CAD build for the part. Positions are in the model's coordinates, mm. A direction names the side the tool comes from. Round coordinates to 2 decimals unless told otherwise and drop trailing zeros. Order: outer loops, then holes, each group sorted by start corner. A loop starts at its lowest first (then second) coordinate and runs counter-clockwise, first axis right, second up.
```python
from build123d import *

# Parameters (mm, degrees)
SKETCH2_W           = 4
SKETCH2_H           = 20
BOSS_EXTRUDE1_DEPTH = 4


with BuildPart() as part:
    # Sketch2 → Boss-Extrude1 (new body)
    with BuildSketch(Plane.XY):
        Polygon((124, 0), (-124, 0), (-129.725981227, -42.426406871), (-120, -42.426406871), (-120, -46.426406871), (-80, -46.426406871), (-80, -42.426406871), (-20, -42.426406871), (-20, -46.426406871), (20, -46.426406871), (20, -42.426406871), (80, -42.426406871), (80, -46.426406871), (120, -46.426406871), (120, -42.426406871), (129.725981227, -42.426406871), align=None)
        with BuildLine():
            Line((-88, -18.534474898), (-88, -8))
            ThreePointArc((-88, -8), (-89.171572875, -5.171572875), (-92, -4))
            Line((-92, -4), (-99.945598546, -4))
            ThreePointArc((-99.945598546, -4), (-103.525730324, -6.215999874), (-103.139076318, -10.408671774))
            Line((-103.139076318, -10.408671774), (-95.193477772, -20.943146672))
            ThreePointArc((-95.193477772, -20.943146672), (-90.729943129, -22.327488943), (-88, -18.534474898))
        make_face(mode=Mode.SUBTRACT)
        with BuildLine():
            Line((-108, -38.426406871), (-100.054401454, -38.426406871))
            ThreePointArc((-100.054401454, -38.426406871), (-96.474269676, -36.210406998), (-96.860923682, -32.017735097))
            Line((-96.860923682, -32.017735097), (-104.806522228, -21.483260199))
            ThreePointArc((-104.806522228, -21.483260199), (-109.270056871, -20.098917928), (-112, -23.891931973))
            Line((-112, -23.891931973), (-112, -34.426406871))
            ThreePointArc((-112, -34.426406871), (-110.828427125, -37.254833996), (-108, -38.426406871))
        make_face(mode=Mode.SUBTRACT)
        with BuildLine():
            Line((-57.139286117, -11.265986324), (-30.309401077, -30.237579974))
            ThreePointArc((-30.309401077, -30.237579974), (-26.161196626, -30.523888986), (-24, -26.971593651))
            Line((-24, -26.971593651), (-24, -8))
            ThreePointArc((-24, -8), (-25.171572875, -5.171572875), (-28, -4))
            Line((-28, -4), (-54.82988504, -4))
            ThreePointArc((-54.82988504, -4), (-58.641967496, -6.788378214), (-57.139286117, -11.265986324))
        make_face(mode=Mode.SUBTRACT)
        with BuildLine():
            Line((-42.860713883, -31.160420547), (-69.690598923, -12.188826897))
            ThreePointArc((-69.690598923, -12.188826897), (-73.838803374, -11.902517885), (-76, -15.454813221))
            Line((-76, -15.454813221), (-76, -34.426406871))
            ThreePointArc((-76, -34.426406871), (-74.828427125, -37.254833996), (-72, -38.426406871))
            Line((-72, -38.426406871), (-45.17011496, -38.426406871))
            ThreePointArc((-45.17011496, -38.426406871), (-41.358032504, -35.638028657), (-42.860713883, -31.160420547))
        make_face(mode=Mode.SUBTRACT)
        with BuildLine():
            Line((3.139076318, -32.017735097), (-4.806522228, -21.483260199))
            ThreePointArc((-4.806522228, -21.483260199), (-9.270056871, -20.098917928), (-12, -23.891931973))
            Line((-12, -23.891931973), (-12, -34.426406871))
            ThreePointArc((-12, -34.426406871), (-10.828427125, -37.254833996), (-8, -38.426406871))
            Line((-8, -38.426406871), (-0.054401454, -38.426406871))
            ThreePointArc((-0.054401454, -38.426406871), (3.525730324, -36.210406998), (3.139076318, -32.017735097))
        make_face(mode=Mode.SUBTRACT)
        with BuildLine():
            Line((12, -18.534474898), (12, -8))
            ThreePointArc((12, -8), (10.828427125, -5.171572875), (8, -4))
            Line((8, -4), (0.054401454, -4))
            ThreePointArc((0.054401454, -4), (-3.525730324, -6.215999874), (-3.139076318, -10.408671774))
            Line((-3.139076318, -10.408671774), (4.806522228, -20.943146672))
            ThreePointArc((4.806522228, -20.943146672), (9.270056871, -22.327488943), (12, -18.534474898))
        make_face(mode=Mode.SUBTRACT)
        with BuildLine():
            Line((112, -23.891931973), (112, -34.426406871))
            ThreePointArc((112, -34.426406871), (110.828427125, -37.254833996), (108, -38.426406871))
            Line((108, -38.426406871), (100.054401454, -38.426406871))
            ThreePointArc((100.054401454, -38.426406871), (96.474269676, -36.210406998), (96.860923682, -32.017735097))
            Line((96.860923682, -32.017735097), (104.806522228, -21.483260199))
            ThreePointArc((104.806522228, -21.483260199), (109.270056871, -20.098917928), (112, -23.891931973))
        make_face(mode=Mode.SUBTRACT)
        with BuildLine():
            Line((103.139076318, -10.408671774), (95.193477772, -20.943146672))
            ThreePointArc((95.193477772, -20.943146672), (90.729943129, -22.327488943), (88, -18.534474898))
            Line((88, -18.534474898), (88, -8))
            ThreePointArc((88, -8), (89.171572875, -5.171572875), (92, -4))
            Line((92, -4), (99.945598546, -4))
            ThreePointArc((99.945598546, -4), (103.525730324, -6.215999874), (103.139076318, -10.408671774))
        make_face(mode=Mode.SUBTRACT)
        with BuildLine():
            Line((28, -4), (54.82988504, -4))
            ThreePointArc((54.82988504, -4), (58.641967496, -6.788378214), (57.139286117, -11.265986324))
            Line((57.139286117, -11.265986324), (30.309401077, -30.237579974))
            ThreePointArc((30.309401077, -30.237579974), (26.161196626, -30.523888986), (24, -26.971593651))
            Line((24, -26.971593651), (24, -8))
            ThreePointArc((24, -8), (25.171572875, -5.171572875), (28, -4))
        make_face(mode=Mode.SUBTRACT)
        with BuildLine():
            Line((72, -38.426406871), (45.17011496, -38.426406871))
            ThreePointArc((45.17011496, -38.426406871), (41.358032504, -35.638028657), (42.860713883, -31.160420547))
            Line((42.860713883, -31.160420547), (69.690598923, -12.188826897))
            ThreePointArc((69.690598923, -12.188826897), (73.838803374, -11.902517885), (76, -15.454813221))
            Line((76, -15.454813221), (76, -34.426406871))
            ThreePointArc((76, -34.426406871), (74.828427125, -37.254833996), (72, -38.426406871))
        make_face(mode=Mode.SUBTRACT)
        with Locations((-118, -21.213203436)):
            Rectangle(SKETCH2_W, SKETCH2_H, mode=Mode.SUBTRACT)
        with Locations((-18, -21.213203436)):
            Rectangle(SKETCH2_W, SKETCH2_H, mode=Mode.SUBTRACT)
        with Locations((-82, -21.213203436)):
            Rectangle(SKETCH2_W, SKETCH2_H, mode=Mode.SUBTRACT)
        with Locations((18, -21.213203436)):
            Rectangle(SKETCH2_W, SKETCH2_H, mode=Mode.SUBTRACT)
        with Locations((82, -21.213203436)):
            Rectangle(SKETCH2_W, SKETCH2_H, mode=Mode.SUBTRACT)
        with Locations((118, -21.213203436)):
            Rectangle(SKETCH2_W, SKETCH2_H, mode=Mode.SUBTRACT)
    extrude(amount=BOSS_EXTRUDE1_DEPTH)


solid = part.part
```
1. Mould opens along Y. For faces 1 (the face through (-76, -25, 2)), 2 (the face through (96.502, -36.266, 1.972)), 3 (the face through (125, -42.426, 2)), 4 (the face through (-20, -44, 2)) say: released by +Y, released by -Y, zero draft, split by the parting line, or undercut.
2. Drill centre lines: line 1 (X direction, y = -42.5, z = 0.9); line 2 (Y direction, x = 97, z = 2.05); line 3 (Y direction, x = 2.5, z = 2.65). Where is each one in solid material? Low to high.
3. Pin check, flat tips, straight feed: P1, Ø1.2, axis at y = -29, z = 1.5, coming from the +X side; P2, Ø2, axis at x = 30.5, z = 3.5, coming from the +Y side; P3, Ø2, axis at x = -37.5, z = 2.5, coming from the -Y side; P4, Ø1.2, axis at y = -45, z = 3, coming from the +X side. Stop position of each tip, or through.
4. Cut at A-A, the plane x = -36.5. Write the cut outline in (y, z), and give its area (3 significant figures).
5. Cut at B-B, the plane z = 3.4. Give the number of separate pieces and of enclosed holes in the cut face, and give its area (3 significant figures).
6. Tool access for faces 5 (the face through (2, 0, 2)), 6 (the face through (-100.78, -26.82, 1.97)): list every direction of +Z, -Z, +X, -X, +Y, -Y with a clear straight run to the whole face (end or side of a thin tool).
Outcome:
1. face 1: undercut
1. face 2: undercut
1. face 3: released by -Y
1. face 4: zero draft
2. line 1: x = -120 to -80, -20 to 20, 80 to 120
2. line 2: y = -46.43 to -37.01, -31.83 to -18.55, -4 to 0
2. line 3: y = -46.43 to -37.5, -31.17 to -17.89, -4 to 0
3. P1: stops at x = 127.99
3. P2: stops at y = 0
3. P3: stops at y = -42.43
3. P4: stops at x = 120
4. outline: (-42.43, 0) - (-25.86, 0) - (-25.86, 4) - (-42.43, 4) - close; (-4, 0) - (0, 0) - (0, 4) - (-4, 4) - close
4. area: 82.3 mm2
5. separate pieces: 1
5. enclosed holes: 16
5. area: 6,970 mm2
6. face 5: +Z, -Z, +X, -X, +Y
6. face 6: +Z, -Z
